```python
from build123d import *

# Parameters (mm, degrees)
SKETCH1_W           = 40
SKETCH1_H           = 16
BOSS_EXTRUDE1_DEPTH = 2
SKETCH2_W           = 40
SKETCH2_H           = 16
SKETCH2_W_2         = 38
SKETCH2_H_2         = 14
BOSS_EXTRUDE2_DEPTH = 2
BOSS_EXTRUDE5_REACH = 45.267
SKETCH3_R           = 2.75
SKETCH4_R           = 1.75
CUT_EXTRUDE1_DEPTH  = 44.266615306
SKETCH5_W           = 5
SKETCH5_H           = 16
BOSS_EXTRUDE6_DEPTH = 16
SKETCH6_W           = 20
SKETCH6_H           = 15
SKETCH6_R           = 2.6
BOSS_EXTRUDE7_DEPTH = 2
SKETCH7_W           = 5
SKETCH7_H           = 1
BOSS_EXTRUDE8_DEPTH = 2
SKETCH9_W           = 11.830057264
SKETCH9_H           = 8
CUT_EXTRUDE3_DEPTH  = 49.795491595
SKETCH10_W          = 5
SKETCH10_H          = 18
BOSS_EXTRUDE9_DEPTH = 14
SKETCH11_W          = 3.17
SKETCH11_H          = 8
CUT_EXTRUDE4_DEPTH  = 49.795491595


with BuildPart() as part:
    # Sketch1 → Boss-Extrude1 (new body)
    with BuildSketch(Plane(origin=(0, 0, 0), x_dir=(1, 0, 0), z_dir=(0, 1, 0))):
        with Locations((20, 8)):
            Rectangle(SKETCH1_W, SKETCH1_H)
    extrude(amount=BOSS_EXTRUDE1_DEPTH)

    # Sketch2 → Boss-Extrude2 (add)
    with BuildSketch(Plane(origin=(0, 2, 0), x_dir=(1, 0, 0), z_dir=(0, 1, 0))):
        with Locations((20, 8)):
            Rectangle(SKETCH2_W, SKETCH2_H)
        with Locations((20, 8)):
            Rectangle(SKETCH2_W_2, SKETCH2_H_2, mode=Mode.SUBTRACT)
    extrude(amount=BOSS_EXTRUDE2_DEPTH)

    # Sketch3 → Boss-Extrude5 (add, up to next)
    with BuildSketch(Plane(origin=(0, 4, 0), x_dir=(1, 0, 0), z_dir=(0, 1, 0)), mode=Mode.PRIVATE) as boss_extrude5_sk1:
        with Locations((17.75, 13.25)):
            Circle(SKETCH3_R)
    boss_extrude5_tool1 = extrude(boss_extrude5_sk1.sketch, amount=-BOSS_EXTRUDE5_REACH, mode=Mode.PRIVATE) - part.part
    # Sketch3 → Boss-Extrude5 (add, up to next)
    with BuildSketch(Plane(origin=(0, 4, 0), x_dir=(1, 0, 0), z_dir=(0, 1, 0)), mode=Mode.PRIVATE) as boss_extrude5_sk2:
        with Locations((36.75, 13.25)):
            Circle(SKETCH3_R)
    boss_extrude5_tool2 = extrude(boss_extrude5_sk2.sketch, amount=-BOSS_EXTRUDE5_REACH, mode=Mode.PRIVATE) - part.part
    add(boss_extrude5_tool1.solids().sort_by_distance((17.75, 4, -13.25))[0])
    add(boss_extrude5_tool2.solids().sort_by_distance((36.75, 4, -13.25))[0])

    # Sketch4 → Cut-Extrude1 (cut, through all)
    with BuildSketch(Plane(origin=(0, 4, 0), x_dir=(1, 0, 0), z_dir=(0, 1, 0))):
        with Locations(Location((17.75, 13.25, 0), (0, 0, 270))):
            Circle(SKETCH4_R)
        with Locations(Location((36.75, 13.25, 0), (0, 0, 270))):
            Circle(SKETCH4_R)
    extrude(amount=-CUT_EXTRUDE1_DEPTH, mode=Mode.SUBTRACT)

    # Sketch5 → Boss-Extrude6 (add)
    with BuildSketch(Plane(origin=(0, 0, 0), x_dir=(-1, 0, 0), z_dir=(0, -1, 0))):
        with Locations((-2.5, 8)):
            Rectangle(SKETCH5_W, SKETCH5_H)
    extrude(amount=BOSS_EXTRUDE6_DEPTH)

    # Sketch6 → Boss-Extrude7 (add)
    # profile 1 of 2: a face of its own
    with BuildSketch(Plane.XZ.offset(16)):
        Polygon((5, -30), (5, 0), (0, 0), (0, -15), (0, -30), align=None)
    # profile 2 of 2: a face of its own
    with BuildSketch(Plane.XZ.offset(16)):
        with Locations((-10, -22.5)):
            Rectangle(SKETCH6_W, SKETCH6_H)
        with Locations(Location((-10, -22.5, 0), (0, 0, 270))):
            Circle(SKETCH6_R, mode=Mode.SUBTRACT)
    extrude(amount=-BOSS_EXTRUDE7_DEPTH)

    # Sketch7 → Boss-Extrude8 (add)
    with BuildSketch(Plane(origin=(0, -14, 0), x_dir=(1, 0, 0), z_dir=(0, 1, 0))):
        with Locations((2.5, 15.5)):
            Rectangle(SKETCH7_W, SKETCH7_H)
    extrude(amount=BOSS_EXTRUDE8_DEPTH)

    # Sketch9 → Cut-Extrude3 (cut, through all)
    with BuildSketch(Plane(origin=(5, 0, 0), x_dir=(0, 0, -1), z_dir=(1, 0, 0))):
        with Locations((5.915028632, -12)):
            Rectangle(SKETCH9_W, SKETCH9_H)
    extrude(amount=-CUT_EXTRUDE3_DEPTH, mode=Mode.SUBTRACT)

    # Sketch10 → Boss-Extrude9 (add)
    with BuildSketch(Plane(origin=(0, 0, -16), x_dir=(-1, 0, 0), z_dir=(0, 0, -1))):
        with Locations((-2.5, -5)):
            Rectangle(SKETCH10_W, SKETCH10_H)
    extrude(amount=BOSS_EXTRUDE9_DEPTH)

    # Sketch11 → Cut-Extrude4 (cut, through all)
    with BuildSketch(Plane(origin=(5, 0, 0), x_dir=(0, 0, -1), z_dir=(1, 0, 0))):
        Polygon((0, -8), (11.830057264, -8), (15.000057264, -8), (15.000057264, -4), (0, -4), align=None)
        with Locations((13.415057264, -12)):
            Rectangle(SKETCH11_W, SKETCH11_H)
    extrude(amount=-CUT_EXTRUDE4_DEPTH, mode=Mode.SUBTRACT)


solid = part.part
```
Design review of the part built by this model. Coordinates are the model's own, in mm. A direction names the side the tool comes from. Coordinates: 2 decimals unless noted, no trailing zeros. Loops run counter-clockwise (first coordinate to the right, second up) from the corner with the lowest first, then second, coordinate; pieces in that order, holes last. Notation, with made-up numbers: (58, 79.25) - (110, 79.25) arc R25 cw to (110, 98.25) - close; hole circle Ø9 at (72, 12). An arc over 180 degrees is marked (long way). Use CSV: the item, a comma, the result in double quotes. Start each with the question number.
1) Consider section D-D on z = -18.25. Write out the cut boundary in (x, y).
2) Consider section B-B on z = -22.5. Write out the cut boundary in (x, y).
3) Consider section C-C on x = 36.75. Write out the cut boundary in (y, z).
4) For pin 1 Ø16.5 at (x, z) = (-10.5, -19.5) entering from +Y; pin 2 Ø2 at (x, y) = (17.5, 3.5) entering from -Z; pin 3 Ø4 at (x, z) = (11, -10.5) entering from -Y, all flat-tipped, find the tip position at first contact; note any pin that passes through.
5) Wall thickness on L1, parallel to X at y = 2.85, z = -13.25; L2, parallel to X at y = 0.9, z = -13.25; L3, parallel to X at y = -15.1, z = -22.5: over which ranges is each line inside the solid? List them lowest first. Write a range as from..to.
6) Consider section A-A on x = -11. Write out the cut boundary in (y, z), then the cut area to 3 significant figures.
7) The part is to be moulded in two halves that separate along X. For faces 5 (the cylindrical face through (19.485, 2.028, -13.478)), 6 (the flat face through (0, -3, -18)), 7 (the flat face through (-2, -15, -15)), say which applies: +X half, -X half, draft (parallel to the pull), parting line (faces both ways), or undercut.
8) Tool access review of faces 1 (the flat face through (23, 2, -16)), 2 (the flat face through (3, -4, -8)), 3 (the flat face through (1, 3, -8)), 4 (the flat face through (22, 0, -8)): name each direction out of +Z, -Z, +X, -X, +Y, -Y from which nothing blocks a thin tool from reaching the whole face with its end or side.
Geometry says:
1,outline,"(-20, -16) - (5, -16) - (5, 4) - (0, 4) - (0, -14) - (-20, -14) - close"
2,outline,"(-20, -16) - (-12.6, -16) - (-12.6, -14) - (-20, -14) - close; (-7.4, -16) - (5, -16) - (5, 4) - (0, 4) - (0, -14) - (-7.4, -14) - close"
3,outline,"(0, -16) - (4, -16) - (4, -15) - (0, -15) - close; (0, -11.5) - (4, -11.5) - (4, -10.5) - (2, -10.5) - (2, -1) - (4, -1) - (4, 0) - (0, 0) - close"
4,pin 1,"y = -14"
4,pin 2,"z = -16"
4,pin 3,"y = 0"
5,L1,"0..1, 15..16, 19.5..20.5, 34..35, 38.5..40"
5,L2,"0..16, 19.5..35, 38.5..40"
5,L3,"-20..-12.6, -7.4..5"
6,outline,"(-16, -30) - (-14, -30) - (-14, -24.9) - (-16, -24.9) - close; (-16, -20.1) - (-14, -20.1) - (-14, -15) - (-16, -15) - close"
6,area,"20.4 mm^2"
7,face 5,"undercut"
7,face 6,"-X half"
7,face 7,"draft"
8,face 1,"-Z, +X, +Y, -Y"
8,face 2,"+Z, +X, -X, -Y"
8,face 3,"+Y"
8,face 4,"+Z, -Z, +X, -Y"
